from build123d import *

# Parameters (mm, degrees)
SKETCH1_W                = 25.4
SKETCH1_H                = 25.4
BOSS_EXTRUDE1_DEPTH      = 200
BOSS_EXTRUDE1_DEPTH_BACK = 200
SKETCH5_R                = 3.2
CUT_EXTRUDE1_DEPTH       = 26.4
SKETCH6_R                = 4
CUT_EXTRUDE2_DEPTH       = 3


with BuildPart() as part:
    # Sketch1 → Boss-Extrude1 (new body, two sides)
    with BuildSketch(Plane.XY) as boss_extrude1_sk:
        Rectangle(SKETCH1_W, SKETCH1_H)
    extrude(amount=BOSS_EXTRUDE1_DEPTH)
    extrude(boss_extrude1_sk.sketch, amount=-BOSS_EXTRUDE1_DEPTH_BACK)

    # Sketch4 → Cut-Revolve1 (revolve, cut)
    with BuildSketch(Plane(origin=(0, 0, 0), x_dir=(0, 0, -1), z_dir=(1, 0, 0))):
        Polygon((-125, -12.7), (-131, -12.7), (-131, 2.3), (-127.75, 4.176388375), (-127.75, 9.7), (-130.55625, 9.7), (-130.55625, 12.7), (-125, 12.7), align=None)
    cut_revolve1 = revolve(axis=Axis((0, 23.510725719, 125), (0, -1, 0)), mode=Mode.SUBTRACT)

    # Mirror1: Cut-Revolve1 across plane
    add(cut_revolve1.mirror(Plane.XY), mode=Mode.SUBTRACT)

    # Sketch5 → Cut-Extrude1 (cut, through all)
    with BuildSketch(Plane(origin=(12.7, 0, 0), x_dir=(0, 0, -1), z_dir=(1, 0, 0))):
        with Locations((-155, 0)):
            Circle(SKETCH5_R)
        with Locations((-95, 0)):
            Circle(SKETCH5_R)
        with Locations((-35, 0)):
            Circle(SKETCH5_R)
        with Locations((35, 0)):
            Circle(SKETCH5_R)
        with Locations((95, 0)):
            Circle(SKETCH5_R)
        with Locations((155, 0)):
            Circle(SKETCH5_R)
    extrude(amount=-CUT_EXTRUDE1_DEPTH, mode=Mode.SUBTRACT)

    # Sketch6 → Cut-Extrude2 (cut)
    with BuildSketch(Plane.ZY.offset(12.7)):
        with Locations((-155, 0)):
            Circle(SKETCH6_R)
        with Locations((-95, 0)):
            Circle(SKETCH6_R)
        with Locations((-35, 0)):
            Circle(SKETCH6_R)
        with Locations((35, 0)):
            Circle(SKETCH6_R)
        with Locations((95, 0)):
            Circle(SKETCH6_R)
        with Locations((155, 0)):
            Circle(SKETCH6_R)
    extrude(amount=-CUT_EXTRUDE2_DEPTH, mode=Mode.SUBTRACT)


solid = part.part
CAD build for the part. Positions are in the model's coordinates, mm. A direction names the side the tool comes from. Give positions to 0.01 mm unless a question says otherwise; leave off trailing zeros. Order: outer loops, then holes, each group sorted by start corner. A loop starts at its lowest first (then second) coordinate and runs counter-clockwise, first axis right, second up. Notation, with made-up numbers: (7.25, -25) -> (14.25, -25) arc R34 ccw to (14.25, 11) -> close; hole circle Ø7 at (65, -5). An arc over 180 degrees is marked (long way). Return JSON: item names as keys, results as strings.
Q1. Mould opens along Y. For faces 1 (the face through (0, 12.7, 3)), 2 (the face through (0, -5, 119)), 3 (the face through (-9.7, 3, -37)) say: pulls with the +Y half, pulls with the -Y half, needs draft (parallel to the pull), parting line crosses it, or undercut.
Working result:
{"face 1": "pulls with the +Y half", "face 2": "needs draft", "face 3": "undercut"}
Q2. Drill centre lines: line 1 (Z direction, x = 0, y = 7.45); line 2 (Y direction, x = -11.7, z = -35); line 3 (X direction, y = -2.75, z = 125). Where is each one in solid material? Low to high.
Working result:
{"line 1": "-200 to -127.75, -122.25 to 122.25, 127.75 to 200", "line 2": "-12.7 to -4, 4 to 12.7", "line 3": "-12.7 to -6, 6 to 12.7"}
Q3. Flat gauge pins, fed straight in: pin 1 (5.5 mm diameter, centred on x = -0.5, z = 124, fed in from +Y); pin 2 (6.5 mm diameter, centred on y = 0, z = -155, fed in from -X). Where does each tip first touch, or does it go through?
Working result:
{"pin 1": "y = 9.7", "pin 2": "x = -9.7"}
Q4. Which spindle directions (+Z, -Z, +X, -X, +Y, -Y) get a long thin tool onto all of the face, cutting with end or side? Do faces 4 (the face through (12.7, 0, 3)), 5 (the face through (1, 9.7, 128)), 6 (the face through (-9.7, 3, -97)). Say none if no direction does.
Working result:
{"face 4": "+Z, -Z, +X, +Y, -Y", "face 5": "+Y", "face 6": "-X"}
Q5. Saw through at A-A (y = -8.5). Write the cut outline in (x, z), then the cut area to 3 significant figures.
Working result:
{"outline": "(-12.7, -200) -> (12.7, -200) -> (12.7, 200) -> (-12.7, 200) -> close; hole circle Ø12 at (0, -125); hole circle Ø12 at (0, 125)", "area": "9,930 mm²"}
